For this review, use the dimensioned drawing (mm, ordinates from the lowest corner) and the shaded views. A direction names the side the tool comes from. Give positions to 0.01 mm unless a question says otherwise; leave off trailing zeros. Loops run counter-clockwise (first coordinate to the right, second up) from the corner with the lowest first, then second, coordinate; pieces in that order, holes last. Notation, with made-up numbers: (74, -2) -> (90, -2) arc R22 cw to (90, 35) -> close; hole circle Ø7 at (83.5, 44). An arc over 180 degrees is marked (long way). Use a Markdown table: item, result. Add a question column.
1. Add section C-C (y = 22.5). State the section outline as (x, z) points.
2. Add section A-A (x = 10.5). State the section outline as (y, z) points.
3. For the marked faces 1, 2 and 3, list the 3-axis set-ups (+Z, -Z, +X, -X, +Y, -Y) from which the entire face can be reached by the end or side of a thin tool; tool diameter is ignored.
4. Add section B-B (z = 39.5). State the section outline as (x, y) points, and give its area (3 significant figures).
5. To check wall thickness, follow line 1 (Y direction, x = 147.5, z = 2.35); line 2 (Z direction, x = 59.5, y = 26); line 3 (Y direction, x = 144.5, z = 40.5). State the ranges of each line that lie inside material, in increasing order.
6. For pin 1 Ø0.6 at (x, y) = (24, 15) entering from +Z; pin 2 Ø1 at (x, y) = (23, 10.5) entering from +Z; pin 3 Ø6 at (x, z) = (46, 89) entering from +Y; pin 4 Ø10 at (y, z) = (7, 77) entering from +X, all flat-tipped, find the tip position at first contact; note any pin that passes through.
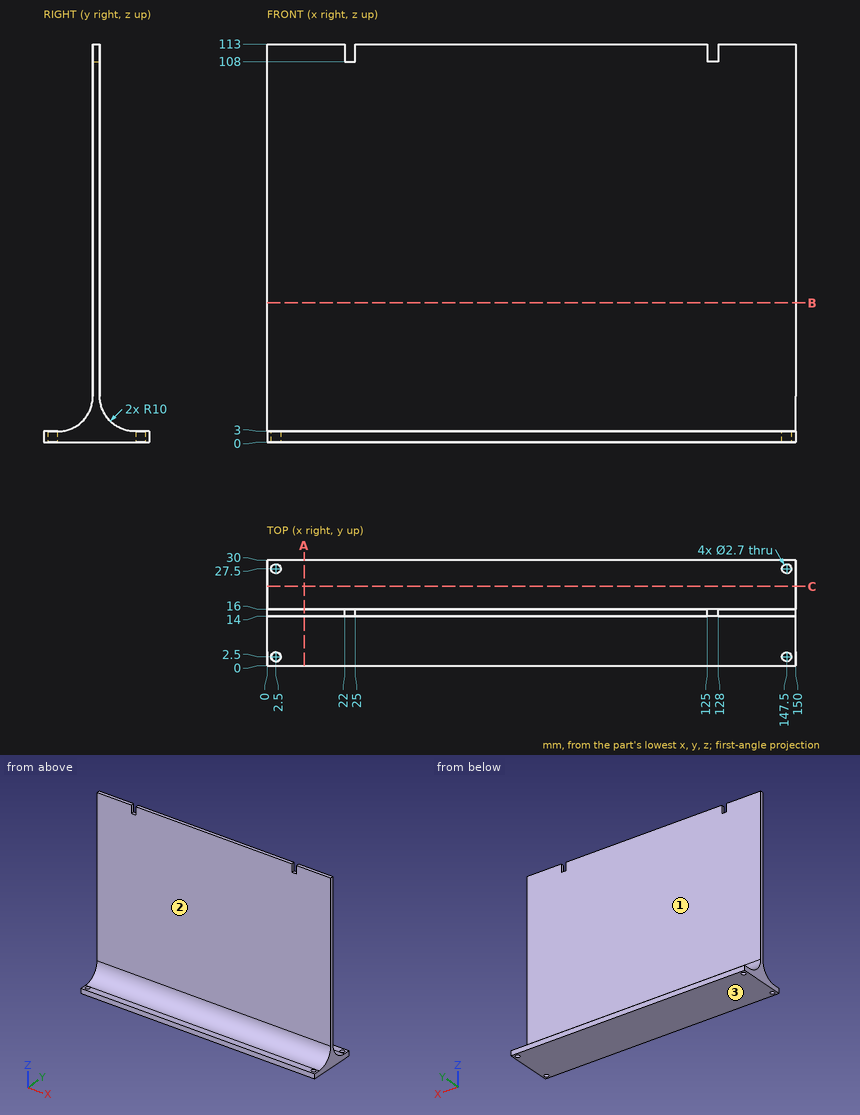
Taken from the geometry:
| question | item | result |
|---|---|---|
| 1 | outline | (0, 0) -> (150, 0) -> (150, 3.63) -> (0, 3.63) -> close |
| 2 | outline | (0, 0) -> (30, 0) -> (30, 3) -> (26, 3) arc R10 cw to (16, 13) -> (16, 113) -> (14, 113) -> (14, 13) arc R10 cw to (4, 3) -> (0, 3) -> close |
| 3 | face 1 | +Z, +X, -X, +Y |
| 3 | face 2 | +Z, +X, -X, -Y |
| 3 | face 3 | -Z, +X, -X, +Y, -Y |
| 4 | outline | (0, 14) -> (150, 14) -> (150, 16) -> (0, 16) -> close |
| 4 | area | 300 mm^2 |
| 5 | line 1 | y = 0 to 1.15, 3.85 to 26.15, 28.85 to 30 |
| 5 | line 2 | z = 0 to 3 |
| 5 | line 3 | y = 14 to 16 |
| 6 | pin 1 | stops at z = 108 |
| 6 | pin 2 | stops at z = 5.86 |
| 6 | pin 3 | stops at y = 16 |
| 6 | pin 4 | passes through |
